Work out the finished part from the listing and answer in its coordinate system (mm). Face numbers are marked on the shaded views. A direction names the side the tool comes from. Coordinates: 2 decimals unless noted, no trailing zeros. Write each loop counter-clockwise with the first axis right and the second up, starting at its lowest first coordinate (ties: lowest second). Pieces come first, ordered by that corner, then holes. Notation, with made-up numbers: (18.5, 89.5) - (64.5, 89.5) arc R30 cw to (64.5, 118.5) - close; hole circle Ø3 at (51.25, 88.5). An arc over 180 degrees is marked (long way). Use a Markdown table: item, result. Add a question column.
(1) The part is cut by section A-A, the plane x = 16. Give the vertices of the cut face in (y, z), then the cut area to 3 significant figures.
(2) Given pin 1 Ø6 at (x, z) = (0, 3.5) entering from -Y; pin 2 Ø3 at (y, z) = (28, 0.5) entering from +X; pin 3 Ø2.5 at (y, z) = (30, 2) entering from +X; pin 4 Ø4 at (y, z) = (28.5, 1.5) entering from -X, each flat-ended and moving along its own axis, determine where each tip first touches the part or whether it passes through.
(3) A tool of negligible diameter and unlimited length cuts with its end or side. For the marked faces 1, 2 and 3, from which of +Z, -Z, +X, -X, +Y, -Y can it reach the whole face along a straight path? Write none if from no direction.
(4) The part is cut by section B-B, the plane y = 25.5. Give the vertices of the cut face in (x, z), then the cut area to 3 significant figures.
(5) Find the intervals of material crossed by line 1 (X direction, y = 4.4, z = -1.5); line 2 (X direction, y = 30, z = -2.75); line 3 (Y direction, x = 14, z = 3.5), in increasing order. Write a range as from..to.
(6) The part is cut by section C-C, the plane x = 3. Give the vertices of the cut face in (y, z), then the cut area to 3 significant figures.
(7) The part is cut by section D-D, the plane z = 4.5. Give the vertices of the cut face in (x, y).
(8) For a pull along X with two mould halves and no side action, classify the marked faces 4, 5, 6 and 7 as released by +X, released by -X, zero draft, split by the parting line, or undercut.
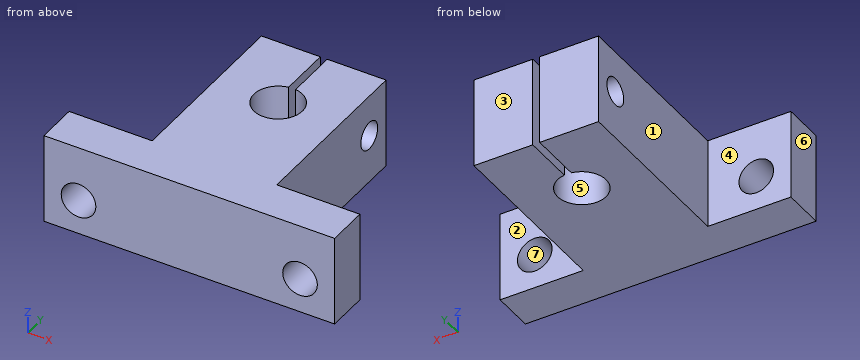
from build123d import *

# Parameters (mm, degrees)
SKETCH1_W           = 42
SKETCH1_H           = 13
SKETCH1_R           = 2.5
BOSS_EXTRUDE1_DEPTH = 6
SKETCH2_W           = 18
SKETCH2_H           = 13
BOSS_EXTRUDE2_DEPTH = 26
SKETCH3_R           = 3.5
CUT_EXTRUDE1_DEPTH  = 26
SKETCH4_R           = 2
CUT_EXTRUDE2_DEPTH  = 26


with BuildPart() as part:
    # Sketch1 → Boss-Extrude1 (new body)
    with BuildSketch(Plane(origin=(0, 0, 0), x_dir=(1, 0, 0), z_dir=(0, 1, 0))):
        Rectangle(SKETCH1_W, SKETCH1_H)
        with Locations(Location((-16, 1.5, 0), (0, 0, 270))):
            Circle(SKETCH1_R, mode=Mode.SUBTRACT)
        with Locations(Location((16, 1.5, 0), (0, 0, 270))):
            Circle(SKETCH1_R, mode=Mode.SUBTRACT)
    extrude(amount=BOSS_EXTRUDE1_DEPTH)

    # Sketch2 → Boss-Extrude2 (add)
    with BuildSketch(Plane(origin=(0, 6, 0), x_dir=(1, 0, 0), z_dir=(0, 1, 0))):
        Rectangle(SKETCH2_W, SKETCH2_H)
    extrude(amount=BOSS_EXTRUDE2_DEPTH)

    # Sketch3 → Cut-Extrude1 (cut)
    with BuildSketch(Plane.XY.offset(6.5)):
        with Locations((0.091950453, 21)):
            Circle(SKETCH3_R)
        with BuildLine():
            Line((0.5, 32), (-0.5, 32))
            Line((-0.5, 32), (-0.5, 24.449578911))
            ThreePointArc((-0.5, 24.449578911), (-0.000953562, 24.49876676), (0.5, 24.476132271))
            Line((0.5, 24.476132271), (0.5, 32))
        make_face()
    extrude(amount=-CUT_EXTRUDE1_DEPTH, mode=Mode.SUBTRACT)

    # Sketch4 → Cut-Extrude2 (cut)
    with BuildSketch(Plane(origin=(9, 0, 0), x_dir=(0, 0, -1), z_dir=(1, 0, 0))):
        with Locations((-0.5, 28)):
            Circle(SKETCH4_R)
    extrude(amount=-CUT_EXTRUDE2_DEPTH, mode=Mode.SUBTRACT)


solid = part.part
Model answer:
| question | item | result |
|---|---|---|
| 1 | outline | (0, -6.5) - (6, -6.5) - (6, -4) - (0, -4) - close; (0, 1) - (6, 1) - (6, 6.5) - (0, 6.5) - close |
| 1 | area | 48.0 mm^2 |
| 2 | pin 1 | y = 0 |
| 2 | pin 2 | through |
| 2 | pin 3 | x = 9 |
| 2 | pin 4 | x = -9 |
| 3 | face 1 | +Z, -Z, -X, +Y |
| 3 | face 2 | +Z, -Z, +X, +Y |
| 3 | face 3 | +Z, -Z, +X, -X, +Y |
| 4 | outline | (-9, -6.5) - (-0.5, -6.5) - (-0.5, 6.5) - (-9, 6.5) - close; (0.5, -6.5) - (9, -6.5) - (9, 6.5) - (0.5, 6.5) - close |
| 4 | area | 221 mm^2 |
| 5 | line 1 | -21..-18.5, -13.5..13.5, 18.5..21 |
| 5 | line 2 | -9..-0.5, 0.5..9 |
| 5 | line 3 | 0..6 |
| 6 | outline | (0, -6.5) - (19.05, -6.5) - (19.05, 6.5) - (0, 6.5) - close; (22.95, -6.5) - (32, -6.5) - (32, 6.5) - (22.95, 6.5) - close; hole circle Ø4 at (28, 0.5) |
| 6 | area | 353 mm^2 |
| 7 | outline | (-21, 0) - (21, 0) - (21, 6) - (9, 6) - (9, 32) - (0.5, 32) - (0.5, 24.48) arc R3.5 cw (long way) to (-0.5, 24.45) - (-0.5, 32) - (-9, 32) - (-9, 6) - (-21, 6) - close |
| 8 | face 4 | zero draft |
| 8 | face 5 | undercut |
| 8 | face 6 | released by -X |
| 8 | face 7 | undercut |
